Geometry: final body of the model. Coordinates: model frame, mm. A direction names the side the tool comes from. Give positions to 0.01 mm unless a question says otherwise; leave off trailing zeros. Loops run counter-clockwise (first coordinate to the right, second up) from the corner with the lowest first, then second, coordinate; pieces in that order, holes last.
from build123d import *

# Parameters (mm, degrees)
SKETCH1_W              = 220
SKETCH1_H              = 260
BOSS_EXTRUDE1_DEPTH    = 20
FILLET1_R              = 30
CUT_EXTRUDE1_START     = -10
CUT_EXTRUDE1_OUTLINE_W = 15
CUT_EXTRUDE1_OUTLINE_H = 20
CUT_EXTRUDE1_DEPTH     = 10
SKETCH8_W              = 15
SKETCH8_H              = 20
CUT_EXTRUDE2_DEPTH     = 10
BOSS_EXTRUDE3_DEPTH    = 10


# Read off the part's stored shape, not the designer's step: Cut-Extrude1
with BuildPart() as part:
    # Sketch1 → Boss-Extrude1 (new body)
    with BuildSketch(Plane(origin=(0, 0, 0), x_dir=(1, 0, 0), z_dir=(0, 1, 0))):
        with Locations((110, 130)):
            Rectangle(SKETCH1_W, SKETCH1_H)
    extrude(amount=BOSS_EXTRUDE1_DEPTH)

    # Fillet1
    fillet1_edges = [part.edges().sort_by_distance(p)[0] for p in [
        (0, 10, -260),
        (220, 10, -260),
        (220, 10, 0),
        (0, 10, 0),
    ]]
    fillet(fillet1_edges, radius=FILLET1_R)

    # Cut-Extrude1 outline → Cut-Extrude1 (cut)
    with BuildSketch(Plane(origin=(220, 0, 0), x_dir=(0, 0, -1), z_dir=(1, 0, 0)).offset(CUT_EXTRUDE1_START)):
        with Locations((232.5, 10)):
            Rectangle(CUT_EXTRUDE1_OUTLINE_W, CUT_EXTRUDE1_OUTLINE_H)
        with Locations((202.5, 10)):
            Rectangle(CUT_EXTRUDE1_OUTLINE_W, CUT_EXTRUDE1_OUTLINE_H)
        with Locations((172.5, 10)):
            Rectangle(CUT_EXTRUDE1_OUTLINE_W, CUT_EXTRUDE1_OUTLINE_H)
        with Locations((142.5, 10)):
            Rectangle(CUT_EXTRUDE1_OUTLINE_W, CUT_EXTRUDE1_OUTLINE_H)
        with Locations((112.5, 10)):
            Rectangle(CUT_EXTRUDE1_OUTLINE_W, CUT_EXTRUDE1_OUTLINE_H)
        with Locations((82.5, 10)):
            Rectangle(CUT_EXTRUDE1_OUTLINE_W, CUT_EXTRUDE1_OUTLINE_H)
        with Locations((52.5, 10)):
            Rectangle(CUT_EXTRUDE1_OUTLINE_W, CUT_EXTRUDE1_OUTLINE_H)
    extrude(amount=CUT_EXTRUDE1_DEPTH, mode=Mode.SUBTRACT)

    # Sketch8 → Cut-Extrude2 (cut)
    with BuildSketch(Plane.ZY):
        with Locations((-222.5, 10)):
            Rectangle(SKETCH8_W, SKETCH8_H)
        with Locations((-192.5, 10)):
            Rectangle(SKETCH8_W, SKETCH8_H)
        with Locations((-162.5, 10)):
            Rectangle(SKETCH8_W, SKETCH8_H)
        with Locations((-132.5, 10)):
            Rectangle(SKETCH8_W, SKETCH8_H)
        with Locations((-102.5, 10)):
            Rectangle(SKETCH8_W, SKETCH8_H)
        with Locations((-72.5, 10)):
            Rectangle(SKETCH8_W, SKETCH8_H)
        with Locations((-42.5, 10)):
            Rectangle(SKETCH8_W, SKETCH8_H)
    extrude(amount=-CUT_EXTRUDE2_DEPTH, mode=Mode.SUBTRACT)

    # Sketch11 → Boss-Extrude3 (add)
    with BuildSketch(Plane.XZ):
        with BuildLine():
            Line((229.686269666, -235), (230, -235))
            Line((230, -235), (230, -30))
            ThreePointArc((230, -30), (218.284271247, -1.715728753), (190, 10))
            Line((190, 10), (30, 10))
            ThreePointArc((30, 10), (1.715728753, -1.715728753), (-10, -30))
            Line((-10, -30), (-10, -225))
            Line((-10, -225), (-9.686269666, -225))
            ThreePointArc((-9.686269666, -225), (0, -256.457513111), (30, -270))
            Line((30, -270), (190, -270))
            ThreePointArc((190, -270), (216.457513111, -260), (229.686269666, -235))
        make_face()
    extrude(amount=BOSS_EXTRUDE3_DEPTH)


solid = part.part
Item 1: Section query A-A on z = -207. Return loops of the section in (x, y).
Values follow:
outline: (-10, -10) - (230, -10) - (230, 0) - (210, 0) - (210, 20) - (0, 20) - (0, 0) - (-10, 0) - close
Item 2: Section query C-C on x = 126. Return loops of the section in (y, z).
Values follow:
outline: (-10, -270) - (0, -270) - (0, -260) - (20, -260) - (20, 0) - (0, 0) - (0, 10) - (-10, 10) - close
Item 3: Set-up query: faces 1 (the face through (8.555, 10.14, -9.021)), 2 (the face through (215, 10, -210)), 3 (the face through (5, 10, -155)). Return all of +Z, -Z, +X, -X, +Y, -Y with unobstructed straight access to the full face (end or side cutting, diameter ignored); none if empty.
Values follow:
face 1: +Z, -X, +Y
face 2: +X, +Y
face 3: -X, +Y
Item 4: Ray query, probe 1 along X at (y, z) = (8.25, -202); probe 2 along X at (y, z) = (4.25, -192); probe 3 along Z at (x, y) = (146, 9.75). Return the intervals inside material, ascending.
Values follow:
probe 1: x = 0 to 210
probe 2: x = 10 to 220
probe 3: z = -260 to 0
Item 5: Section query B-B on y = -3.75. Return loops of the section in (x, z), plus the area to 3 significant figures.
Values follow:
outline: (-10, -225) - (-9.69, -225) arc R40 ccw to (30, -270) - (190, -270) arc R40 ccw to (229.69, -235) - (230, -235) - (230, -30) arc R40 ccw to (190, 10) - (30, 10) arc R40 ccw to (-10, -30) - close
area: 65,800 mm2
Item 6: Pin query (flat end, axial travel): pin 1 (6 mm diameter, centred on x = 84.5, y = 11, fed in from +Z); pin 2 (3 mm diameter, centred on x = 3, y = 13.5, fed in from +Z); pin 3 (5 mm diameter, centred on x = 4, y = 13, fed in from -Z); pin 4 (10 mm diameter, centred on y = 0.5, z = -72, fed in from -X). Return the tip coordinate at first contact, or that it passes through.
Values follow:
pin 1: stops at z = 0
pin 2: stops at z = -14.2
pin 3: stops at z = -248.65
pin 4: stops at x = -10
Item 7: Draft query along Z for faces 4 (the face through (10, 10, -223)), 5 (the face through (208, 10, -254)), 6 (the face through (218.594, -4.93, -2.028)), 7 (the face through (0, 10, -57)). Return one class per face: +Z half, -Z half, draft (parallel to the pull), parting line (faces both ways), or undercut.
Values follow:
face 4: undercut
face 5: -Z half
face 6: +Z half
face 7: draft
